Study the drawing (mm; zero at the part's minimum x, y, z) and answer. A direction names the side the tool comes from. Give positions to 0.01 mm unless a question says otherwise; leave off trailing zeros. Write each loop counter-clockwise with the first axis right and the second up, starting at its lowest first coordinate (ties: lowest second). Pieces come first, ordered by that corner, then holes. Notation, with made-up numbers: (87.5, 53) - (142.5, 53) arc R18 ccw to (142.5, 74) - close; hole circle Ø10 at (36, 48). An arc over 180 degrees is marked (long way). Return JSON: item names as keys, results as strings.
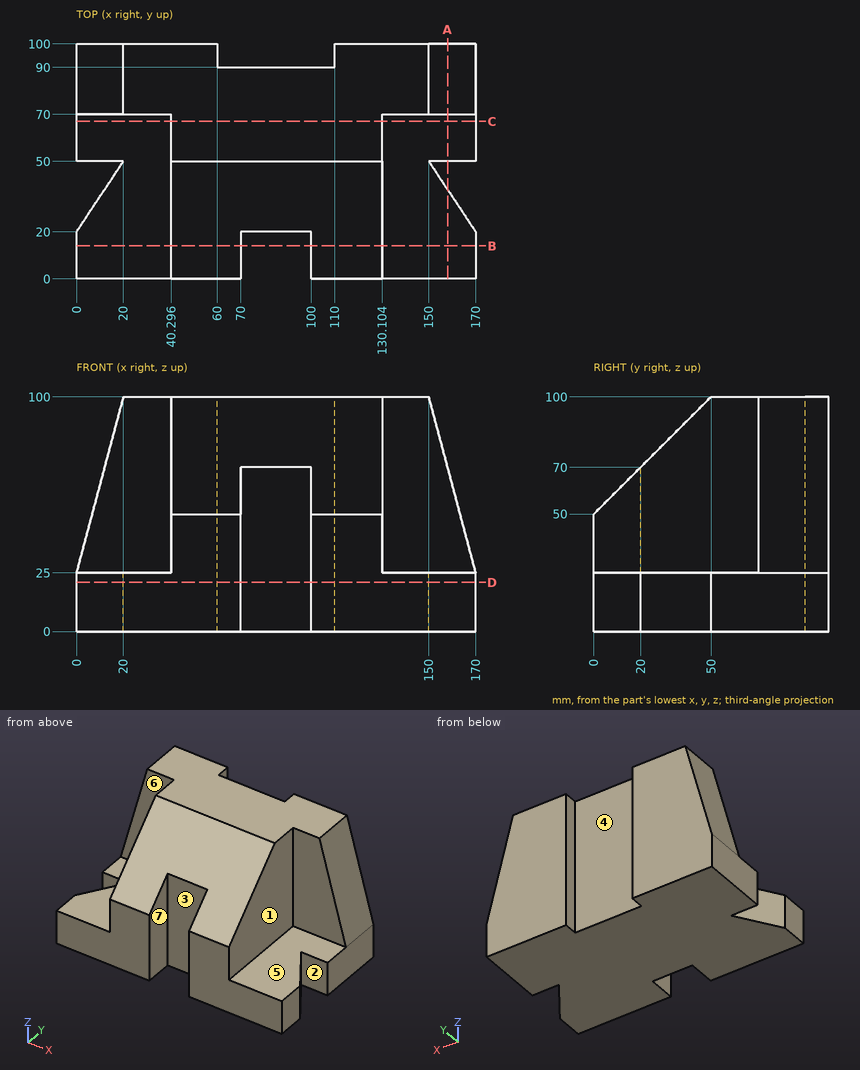
Item 1: A cutting plane is placed at C-C on y = 67. Determine the outline of the cut face in (x, z) (1 decimal), then the cut area to 3 significant figures.
Answer below:
{"outline": "(0, 0) - (170, 0) - (170, 25) - (130.1, 25) - (130.1, 100) - (40.3, 100) - (40.3, 25) - (0, 25) - close", "area": "11,000 mm²"}
Item 2: Consider L1, parallel to X at y = 9, z = 8; L2, parallel to X at y = 17.5, z = 64.5 (1 decimal); L3, parallel to X at y = 62, z = 82.5 (1 decimal). Determine where each line is inside the solid, lowest interval first.
Answer below:
{"L1": "x = 0 to 70, 100 to 170", "L2": "x = 40.3 to 70, 100 to 130.1", "L3": "x = 40.3 to 130.1"}
Item 3: A cutting plane is placed at D-D on z = 21. Determine the outline of the cut face in (x, y), then the cut area to 3 significant figures.
Answer below:
{"outline": "(0, 0) - (70, 0) - (70, 20) - (100, 20) - (100, 0) - (170, 0) - (170, 20) - (150, 50) - (170, 50) - (170, 100) - (110, 100) - (110, 90) - (60, 90) - (60, 100) - (0, 100) - (0, 50) - (20, 50) - (0, 20) - close", "area": "15,300 mm²"}
Item 4: For the marked faces 5, 6 and 7, determine the directions among +Z, -Z, +X, -X, +Y, -Y from which every point of the face is accessible in a straight line to the end or side of a thin tool.
Answer below:
{"face 5": "+Z, +X, -Y", "face 6": "+Z, -X, -Y", "face 7": "+Z, -Z, -Y"}
Item 5: A cutting plane is placed at B-B on y = 14. Determine the outline of the cut face in (x, z) (1 decimal), then the cut area to 3 significant figures.
Answer below:
{"outline": "(0, 0) - (70, 0) - (70, 64) - (40.3, 64) - (40.3, 25) - (0, 25) - close; (100, 0) - (170, 0) - (170, 25) - (130.1, 25) - (130.1, 64) - (100, 64) - close", "area": "5,830 mm²"}
Item 6: A cutting plane is placed at A-A on x = 158. Determine the outline of the cut face in (y, z).
Answer below:
{"outline": "(0, 0) - (38, 0) - (38, 25) - (0, 25) - close; (50, 0) - (100, 0) - (100, 70) - (70, 70) - (70, 25) - (50, 25) - close"}
Item 7: Flat-ended cylindrical pins translate along their axes: P1, Ø20, axis at x = 25.5, y = 26, coming from the +Z side; P2, Ø11, axis at y = 93.5, z = 47.5, coming from the -X side; P3, Ø3, axis at y = 12, z = 29, coming from the +X side. Find the tip coordinate at first contact, or state that the pin passes through.
Answer below:
{"P1": "stops at z = 25", "P2": "stops at x = 4.53", "P3": "stops at x = 130.1"}
Item 8: The mould has two halves that part along Y. Classify the marked faces 1, 2, 3 and 4: +Y half, -Y half, draft (parallel to the pull), parting line (faces both ways), or undercut.
Answer below:
{"face 1": "draft", "face 2": "undercut", "face 3": "-Y half", "face 4": "+Y half"}
